```python
from build123d import *

# Parameters (mm, degrees)
SKETCH1_W           = 80
SKETCH1_H           = 76.35
SKETCH1_R           = 1.75
SKETCH1_R_2         = 12.25
SKETCH1_R_3         = 2.15
BOSS_EXTRUDE1_DEPTH = 3.175


with BuildPart() as part:
    # Sketch1 → Boss-Extrude1 (new body)
    with BuildSketch(Plane.XY):
        Rectangle(SKETCH1_W, SKETCH1_H)
        with Locations((0, 20)):
            Circle(SKETCH1_R, mode=Mode.SUBTRACT)
        Circle(SKETCH1_R_2, mode=Mode.SUBTRACT)
        with Locations((17.320508076, -10)):
            Circle(SKETCH1_R, mode=Mode.SUBTRACT)
        with Locations((-17.320508076, -10)):
            Circle(SKETCH1_R, mode=Mode.SUBTRACT)
        with Locations((-32, 24.2)):
            Circle(SKETCH1_R_3, mode=Mode.SUBTRACT)
        with Locations(Location((32, 24.2, 0), (0, 0, 180))):
            Circle(SKETCH1_R_3, mode=Mode.SUBTRACT)
        with Locations((32, -24.2)):
            Circle(SKETCH1_R_3, mode=Mode.SUBTRACT)
        with Locations(Location((-32, -24.2, 0), (0, 0, 180))):
            Circle(SKETCH1_R_3, mode=Mode.SUBTRACT)
    extrude(amount=BOSS_EXTRUDE1_DEPTH)


solid = part.part
```
Build history of the part. All positions in model axes, mm. Round coordinates to 2 decimals unless told otherwise and drop trailing zeros. Write each loop counter-clockwise with the first axis right and the second up, starting at its lowest first coordinate (ties: lowest second). Pieces come first, ordered by that corner, then holes. Notation, with made-up numbers: (-15, -3) - (13, -3) arc R35 ccw to (13, 34) - close; hole circle Ø1 at (82, 63.25). An arc over 180 degrees is marked (long way). Write each question's results on one line, items separated by ' | '. Start each with the question number.
Item 1: Mould opens along X. For faces 1 (the face through (-1, -38.175, 2)), 2 (the face through (-40, -1, 2)), 3 (the face through (-0.228, 21.735, 1.565)) say: pulls with the +X half, pulls with the -X half, needs draft (parallel to the pull), parting line crosses it, or undercut.
Item 2: Saw through at A-A (x = 32). Write the cut outline in (y, z) (3 decimals), and give its area (3 significant figures).
Item 3: Saw through at D-D (y = -24.2). Write the cut outline in (x, z) (3 decimals).
Item 4: Saw through at B-B (y = 0). Write the cut outline in (x, z) (3 decimals).
Item 5: Wall check: L1, parallel to Y at x = -32, z = 1.4 (3 decimals); L2, parallel to Y at x = 0, z = 1.1 (3 decimals); L3, parallel to X at y = -9, z = 2.45. Give the ranges that are in metal, low to high. Write a range as [from, to].
Item 6: Saw through at C-C (z = 1.3). State how many separate pieces and enclosed holes the cut face has, and give its area (3 significant figures).
Results are:
1) face 1: needs draft | face 2: pulls with the -X half | face 3: undercut
2) outline: (-38.175, 0) - (-26.35, 0) - (-26.35, 3.175) - (-38.175, 3.175) - close; (-22.05, 0) - (22.05, 0) - (22.05, 3.175) - (-22.05, 3.175) - close; (26.35, 0) - (38.175, 0) - (38.175, 3.175) - (26.35, 3.175) - close | area: 215 mm²
3) outline: (-40, 0) - (-34.15, 0) - (-34.15, 3.175) - (-40, 3.175) - close; (-29.85, 0) - (29.85, 0) - (29.85, 3.175) - (-29.85, 3.175) - close; (34.15, 0) - (40, 0) - (40, 3.175) - (34.15, 3.175) - close
4) outline: (-40, 0) - (-12.25, 0) - (-12.25, 3.175) - (-40, 3.175) - close; (12.25, 0) - (40, 0) - (40, 3.175) - (12.25, 3.175) - close
5) L1: y = [-38.175, -26.35], [-22.05, 22.05], [26.35, 38.175] | L2: y = [-38.175, -12.25], [12.25, 18.25], [21.75, 38.175] | L3: x = [-40, -18.76], [-15.88, -8.31], [8.31, 15.88], [18.76, 40]
6) separate pieces: 1 | enclosed holes: 8 | area: 5,550 mm²
